Read the model definition and answer for the solid it produces. Units are mm, in the model's axes. Face numbers are marked on the shaded views. Give positions to 0.01 mm unless a question says otherwise; leave off trailing zeros. Order: outer loops, then holes, each group sorted by start corner. A loop starts at its lowest first (then second) coordinate and runs counter-clockwise, first axis right, second up. Notation, with made-up numbers: (-25.75, 45) -> (-2.75, 45) arc R21 cw to (-2.75, 56) -> close; hole circle Ø2 at (77, -0.5). An arc over 180 degrees is marked (long way). Use one line per item in the form item = value.
```python
from build123d import *

# Parameters (mm, degrees)
F1_DEPTH  = 12.7
F3_DEPTH  = 2.54
F5_D      = 5.1054
F7_D      = 4.0386
F9_D      = 5.1054
F10_R     = 2.38125
F11_DEPTH = 12.701
F12_R     = 6.35
F13_R     = 5.08


with BuildPart() as f1:
    # F0 (on Top) → F1 (new body)
    with BuildSketch(Plane.XY):
        Polygon((41.275, 41.275), (41.275, 60.325), (-60.325, 60.325), (-60.325, -60.325), (60.325, -60.325), (60.325, 41.275), align=None)
    extrude(amount=F1_DEPTH)

    # F2 (on face) → F3 (cut)
    with BuildSketch(Plane.XY.offset(12.7)):
        Polygon((0.4572, 60.325), (-19.5072, 60.325), (-19.5072, -19.5072), (60.325, -19.5072), (60.325, 0.4572), (0.4572, 0.4572), align=None)
    extrude(amount=-F3_DEPTH, mode=Mode.SUBTRACT)

    # F5 (through all)
    with Locations(Plane(origin=(0, 0, 0), x_dir=(1, 0, 0), z_dir=(0, 0, -1))):
        with Locations((-41.275, -41.275), (22.225, -41.275), (41.275, -22.225), (41.275, 41.275), (-22.225, 41.275), (-41.275, 22.225)):
            Hole(F5_D / 2)

    # F7 (through all)
    with Locations(Plane.XY.offset(12.7)):
        with Locations((4.2672, 15.875), (-23.3172, 15.875), (15.875, 4.2672), (15.875, -23.3172)):
            Hole(F7_D / 2)

    # F9 (through all)
    with Locations(Plane(origin=(0, 0, 0), x_dir=(1, 0, 0), z_dir=(0, 0, -1))):
        with Locations((-41.275, 41.275)):
            Hole(F9_D / 2)

    # F10 (on face) → F11 (cut, through all)
    with BuildSketch(Plane(origin=(0, 0, 0), x_dir=(1, 0, 0), z_dir=(0, 0, -1))):
        with Locations((9.525, 41.275)):
            Circle(F10_R)
        with Locations((41.275, -9.525)):
            Circle(F10_R)
        with Locations((9.525, -41.275)):
            Circle(F10_R)
        with Locations((-41.275, -9.525)):
            Circle(F10_R)
    extrude(amount=-F11_DEPTH, mode=Mode.SUBTRACT)

    # F12
    f12_edges = [f1.edges().sort_by_distance(p)[0] for p in [
        (-19.5072, -19.5072, 11.43),
    ]]
    fillet(f12_edges, radius=F12_R)

    # F13
    f13_edges = [f1.edges().sort_by_distance(p)[0] for p in [
        (-60.325, -60.325, 6.35),
    ]]
    fillet(f13_edges, radius=F13_R)


solid = f1.part
```
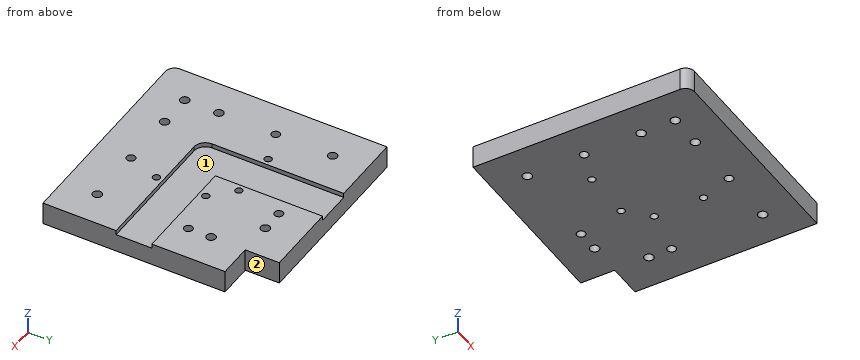
Item 1: The part is cut by section D-D on x = -9. Give the vertices of the cut face in (y, z) (3 decimals).
Checks:
outline = (-60.325, 0) -> (60.325, 0) -> (60.325, 10.16) -> (-19.507, 10.16) -> (-19.507, 12.7) -> (-60.325, 12.7) -> close
Item 2: Given pin 1 Ø3 at (x, y) = (-41.275, 41.275) entering from -Z, flat-ended and moving along its own axis, determine where the tip first touches the part or whether it passes through.
Checks:
pin_1 = through
Item 3: Determine the mould class of the marked faces 1 and 2 for opening direction Y: +Y half, -Y half, draft (parallel to the pull), parting line (faces both ways), or undercut.
Checks:
face_1 = undercut
face_2 = draft
Item 4: The part is cut by section C-C on z = 5.5. State how many separate pieces and enclosed holes the cut face has, and give its area (3 significant figures).
Checks:
separate_pieces = 1
enclosed_holes = 15
area = 13,900 mm²
Item 5: Straight lines are drawn through the part: L1, parallel to Y at x = 9.5, z = 5.5 (3 decimals); L2, parallel to Y at x = 43, z = 10.25 (3 decimals); L3, parallel to Y at x = -22, z = 11 (3 decimals). For each, find the intervals that lie inside material, in ascending order. Write a range as from..to.
Checks:
L1 = -60.325..-43.656, -38.894..38.894, 43.656..60.325
L2 = -60.325..-43.157, -39.393..-19.507, 0.457..7.883, 11.167..20.343, 24.107..41.275
L3 = -60.325..-43.818, -38.732..14.344, 17.406..60.325
Item 6: The part is cut by section A-A on x = 29. Give the vertices of the cut face in (y, z) (3 decimals).
Checks:
outline = (-60.325, 0) -> (60.325, 0) -> (60.325, 12.7) -> (0.457, 12.7) -> (0.457, 10.16) -> (-19.507, 10.16) -> (-19.507, 12.7) -> (-60.325, 12.7) -> close
